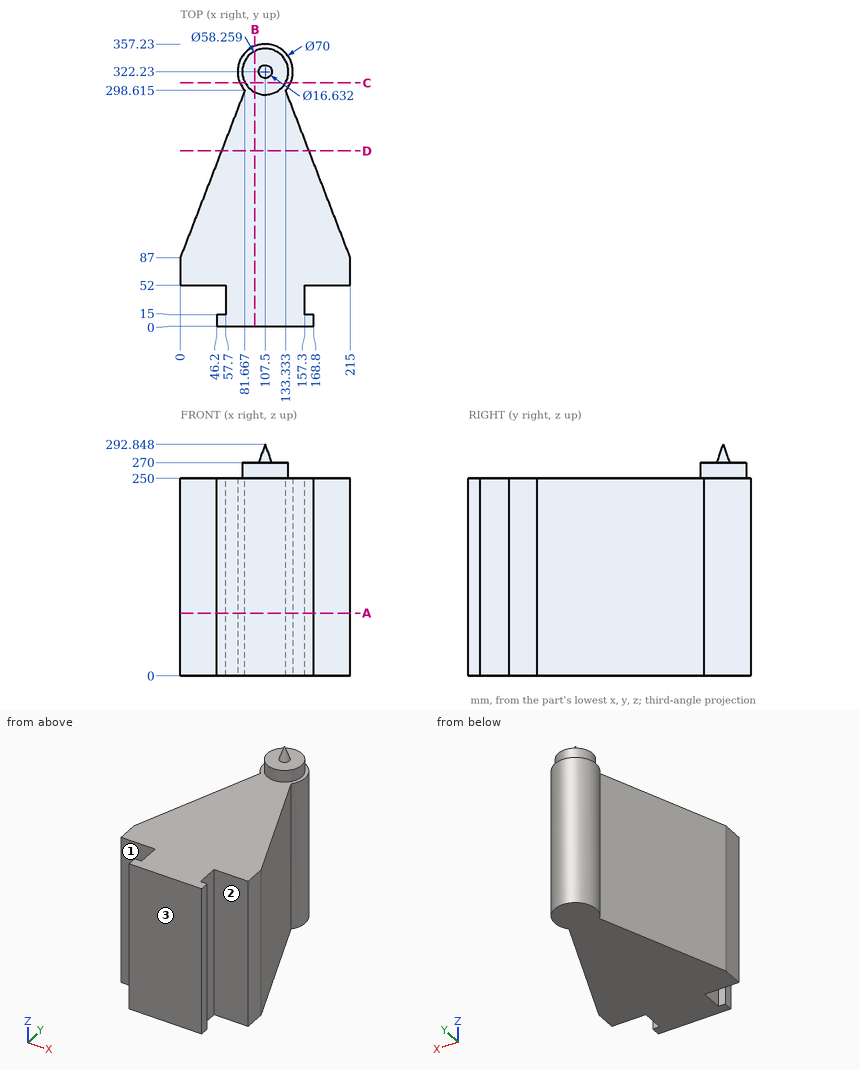
Study the drawing (mm; zero at the part's minimum x, y, z) and answer. A direction names the side the tool comes from. Coordinates: 2 decimals unless noted, no trailing zeros. Write each loop counter-clockwise with the first axis right and the second up, starting at its lowest first coordinate (ties: lowest second). Pieces come first, ordered by that corner, then holes. Notation, with made-up numbers: M 74.25,-11.75 L 121.25,-11.75 A28 cw 121.25,26.25 Z; hole C 64,13.5 d8. An arc over 180 degrees is marked long. Use a Markdown table: item, result. Add a question column.
1. Section D-D (y = 222) is taken. Give the vertices of the cut face in (x, z).
2. Which of the six approach directions +Z, -Z, +X, -X, +Y, -Y give full straight-line access (tool end or side, diameter ignored) to the marked faces 1, 2 and 3?
3. Given P1, Ø11, axis at y = 41.5, z = 120, coming from the -X side; P2, Ø1, axis at y = 229, z = 145, coming from the +X side; P3, Ø6, axis at y = 169, z = 105.5, coming from the -X side, each flat-ended and moving along its own axis, determine where each tip first touches the part or whether it passes through.
4. Section C-C (y = 308) is taken. Give the vertices of the cut face in (x, z), plus the area to 3 significant figures.
5. Straight lines are drawn through the part: line 1 along X through (y, z) = (320, 183); line 2 along Z through (x, y) = (127, 236.5); line 3 along X through (y, z) = (148, 147). For each, find the intervals that lie inside material, in ascending order. Write a range as [from, to].
6. Section B-B (x = 94.5) is taken. Give the vertices of the cut face in (y, z), plus the area to 3 significant figures.
7. Section A-A (z = 79.5) is taken. Give the vertices of the cut face in (x, y) (3 decimals).
Data:
| question | item | result |
|---|---|---|
| 1 | outline | M 52.1,0 L 162.9,0 L 162.9,250 L 52.1,250 Z |
| 2 | face 1 | +Z, -Z, -X |
| 2 | face 2 | +Z, -Z, +X |
| 2 | face 3 | +Z, -Z, +X, -X, -Y |
| 3 | P1 | stops at x = 57.7 |
| 3 | P2 | stops at x = 160.39 |
| 3 | P3 | stops at x = 30.49 |
| 4 | outline | M 75.52,0 L 139.48,0 L 139.48,250 L 132.92,250 L 132.92,270 L 82.08,270 L 82.08,250 L 75.52,250 Z |
| 4 | area | 17,000 mm2 |
| 5 | line 1 | x = [72.57, 142.43] |
| 5 | line 2 | z = [0, 250] |
| 5 | line 3 | x = [23.54, 191.46] |
| 6 | outline | M 0,0 L 354.73,0 L 354.73,250 L 348.3,250 L 348.3,270 L 296.16,270 L 296.16,250 L 0,250 Z |
| 6 | area | 89,700 mm2 |
| 7 | outline | M 0,52 L 57.7,52 L 57.7,15 L 46.2,15 L 46.2,0 L 168.8,0 L 168.8,15 L 157.3,15 L 157.3,52 L 215,52 L 215,87 L 133.333,298.615 A35 ccw long 81.667,298.615 L 0,87 Z |
